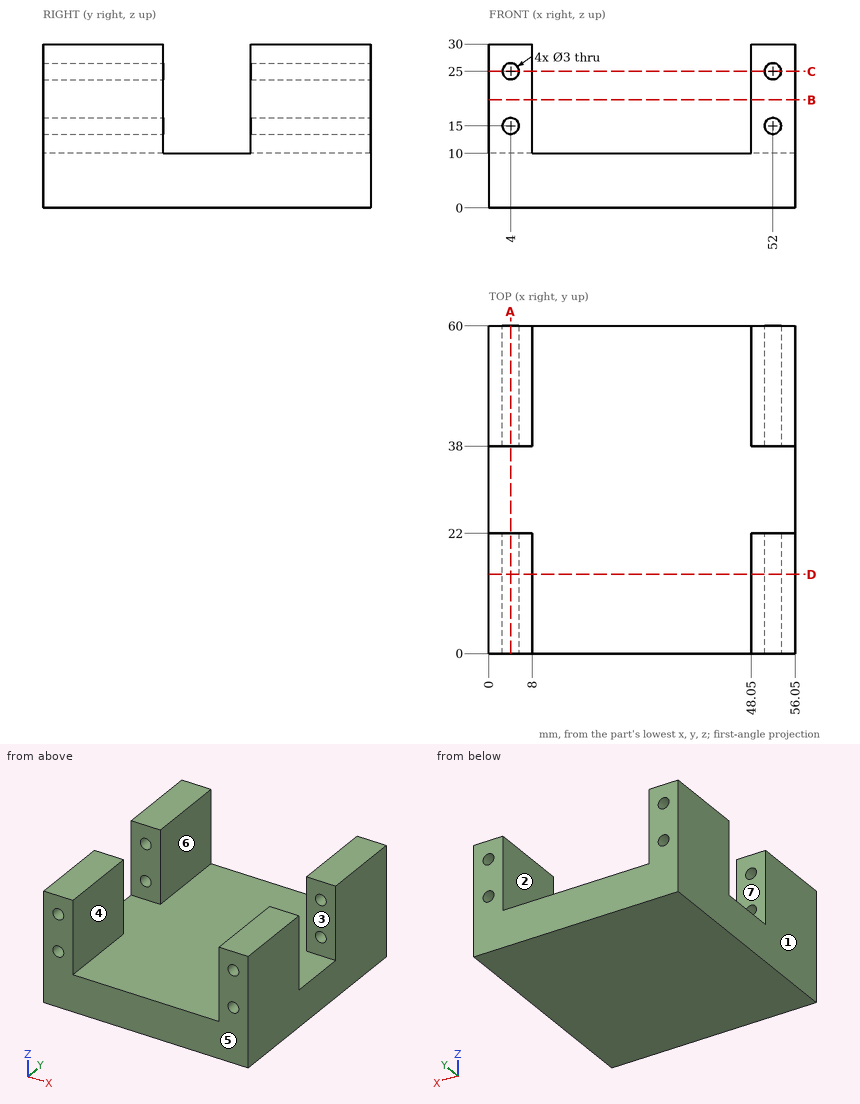
Here's the drawing with two shaded views (mm, measured from the low corner). I have some questions. A direction names the side the tool comes from. Coordinates: 2 decimals unless noted, no trailing zeros. Write each loop counter-clockwise with the first axis right and the second up, starting at its lowest first coordinate (ties: lowest second). Pieces come first, ordered by that corner, then holes. Notation, with made-up numbers: (79.5, -40) -> (114.5, -40) arc R19 cw to (114.5, -25) -> close; hole circle Ø9 at (49, 24.5). An arc over 180 degrees is marked (long way). Use a Markdown table: item, result. Add a question column.
(1) If we section it at B-B, the plane z = 19.75: Write out the boundary of the cut face in (x, y), and give its area (3 significant figures).
(2) If we section it at A-A, the plane x = 4: Write out the boundary of the cut face in (y, z), and give its area (3 significant figures).
(3) For the marked faces 5, 6 and 7, which set-ups out of +Z, -Z, +X, -X, +Y, -Y let a thin tool reach every point of the face, with its end or its side?
(4) If we section it at C-C, the plane z = 25: State how many separate pieces and enclosed holes the cut face has, and give its area (3 significant figures).
(5) If we section it at D-D, the plane y = 14.5: Write out the boundary of the cut face in (x, z), and give its area (3 significant figures).
(6) Please list where these lines run through material, in increasing order: line 1 (Z direction, x = 52, y = 6.5); line 2 (X direction, y = 45.25, z = 25); line 3 (X direction, y = 3.5, z = 28.5).
(7) I'm going to push flat-ended pins straight in: P1, Ø2.5, axis at x = 51, z = 22, coming from the -Y side; P2, Ø1, axis at x = 12, y = 22, coming from the +Z side. Where does each tip first touch, or does it pass through?
(8) We'd pull the mould along X, two halves only. Please class the marked faces 1, 2, 3 and 4: +X half, -X half, draft (parallel to the pull), parting line (faces both ways), or undercut.
Outcome:
| question | item | result |
|---|---|---|
| 1 | outline | (0, 0) -> (8, 0) -> (8, 22) -> (0, 22) -> close; (0, 38) -> (8, 38) -> (8, 60) -> (0, 60) -> close; (48.05, 0) -> (56.05, 0) -> (56.05, 22) -> (48.05, 22) -> close; (48.05, 38) -> (56.05, 38) -> (56.05, 60) -> (48.05, 60) -> close |
| 1 | area | 704 mm^2 |
| 2 | outline | (0, 0) -> (60, 0) -> (60, 13.5) -> (38, 13.5) -> (38, 10) -> (22, 10) -> (22, 13.5) -> (0, 13.5) -> close; (0, 16.5) -> (22, 16.5) -> (22, 23.5) -> (0, 23.5) -> close; (0, 26.5) -> (22, 26.5) -> (22, 30) -> (0, 30) -> close; (38, 16.5) -> (60, 16.5) -> (60, 23.5) -> (38, 23.5) -> close; (38, 26.5) -> (60, 26.5) -> (60, 30) -> (38, 30) -> close |
| 2 | area | 1,220 mm^2 |
| 3 | face 5 | +Z, -Z, +X, -X, -Y |
| 3 | face 6 | +Z, +Y, -Y |
| 3 | face 7 | +Z, +X, -X |
| 4 | separate pieces | 8 |
| 4 | enclosed holes | 0 |
| 4 | area | 440 mm^2 |
| 5 | outline | (0, 0) -> (56.05, 0) -> (56.05, 30) -> (48.05, 30) -> (48.05, 10) -> (8, 10) -> (8, 30) -> (0, 30) -> close; hole circle Ø3 at (4, 15); hole circle Ø3 at (4, 25); hole circle Ø3 at (52, 15); hole circle Ø3 at (52, 25) |
| 5 | area | 852 mm^2 |
| 6 | line 1 | z = 0 to 13.5, 16.5 to 23.5, 26.5 to 30 |
| 6 | line 2 | x = 0 to 2.5, 5.5 to 8, 48.05 to 50.5, 53.5 to 56.05 |
| 6 | line 3 | x = 0 to 8, 48.05 to 56.05 |
| 7 | P1 | stops at y = 0 |
| 7 | P2 | stops at z = 10 |
| 8 | face 1 | -X half |
| 8 | face 2 | undercut |
| 8 | face 3 | draft |
| 8 | face 4 | undercut |
